Source: CAD feature listing. Evaluate the final solid. Frame: model axes, mm. A direction names the side the tool comes from. Round coordinates to 2 decimals unless told otherwise and drop trailing zeros. Order: outer loops, then holes, each group sorted by start corner. A loop starts at its lowest first (then second) coordinate and runs counter-clockwise, first axis right, second up. Notation, with made-up numbers: (55.5, 10) -> (105.5, 10) arc R16 ccw to (105.5, 30) -> close; hole circle Ø2 at (64.25, -7). An arc over 180 degrees is marked (long way). Write item = value, one per line. Start each with the question number.
(1) Ray query, line 1 (X direction, y = 0.05, z = 0); line 2 (Y direction, x = 2.25, z = 6.5). Return the intervals inside material, ascending.
(2) Reachability of faces 1 (the face through (-6, 14.15, -3)), 2 (the face through (-1.398, 3.549, 6.297)), 3 (the face through (1, -2, -3)) from +Z, -Z, +X, -X, +Y, -Y: full face, straight path, thin tool, end or side. Return the list, or none.
(3) Contact query for flat-ended pins moving along their axis: pin 1 Ø2 at (x, y) = (4, 14.5) entering from -Z; pin 2 Ø6 at (y, z) = (5.5, 4.5) entering from +X; pin 3 Ø1 at (y, z) = (3, -4.5) entering from +X. Output: stop coordinate, or through.
(4) Cut plane A-A on y = 12.5. Return the cut outline in (x, z), then the cut area to 3 significant figures.
(5) Draft query along X for faces 4 (the face through (2.111, -1.875, 4.059)), 5 (the face through (-0.35, 8.87, 1.56)), 6 (the face through (3, 7, -6)). Return one class per face: released by +X, released by -X, zero draft, split by the parting line, or undercut.
(6) Cut plane B-B on y = 9.25. Return the cut outline in (x, z).
Autodesk Inventor part; units mm, degrees
ref_plane "YZ Plane" through (0, 0, 0) normal (1, 0, 0) x (0, 1, 0)
ref_plane "XZ Plane" through (0, 0, 0) normal (0, 1, 0) x (-1, 0, 0)
ref_plane "XY Plane" through (0, 0, 0) normal (0, 0, 1) x (1, 0, 0)
sketch "Sketch1" plane through (0, 0, 0) normal (0, 0, 1) x (1, 0, 0)
  line L0 (0, 0) -> (0, 8.9988) construction
  line L1 (0, 0) -> (7.1408, 0) construction
  line L2 (0.9, 0) -> (2.3166, 18)
  line L3 (0.9, 0) -> (6.45, 0)
  line L4 (6.45, 0) -> (6.45, 7)
  line L5 (6.45, 7) -> (8, 7)
  line L6 (6.5, 18) -> (2.3166, 18)
  line L7 (6.5, 18) -> (5.85, 18)
  line L8 (5.85, 18) -> (5.85, 15)
  line L9 (5.85, 15) -> (6.5, 15)
  line L10 (6.5, 15) -> (6.5, 18)
  line L11 (5.85, 16.45) -> (5.3, 18)
  circle A0 centre (6.5, 15) radius 0.85
  line L12 (8, 7) -> (8, 14.15)
  line L13 (8, 14.15) -> (6.5, 14.15)
  line L14 (6.5, 14.15) -> (6.5, 15)
  point P0 (5.85, 15.5477)
  point P1 (6.5, 14.15)
  dimension "d0" = 7
  dimension "d1" = 6.45
  dimension "d4" = 18
  dimension "d6" = 4.5
  dimension "d7" = 0.9
  dimension "d9" = 1.7
  dimension "d10" = 3
  dimension "d11" = 0.55
  dimension "d12" = 1.55
  dimension "d18" = 6.5
  dimension "d19" = 0.65
  dimension "d20" = 8
revolve "Revolution1" add sketch "Sketch1" angle 360 about axis through (0, 0, 0) along (0, 1, 0) contours L2 L6 L11 L8 A0 L13 L12 L5 L4 L3
chamfer "Chamfer1" distance 0.5 angle 45 3 edges at (-8, 7, 0) (-2.3166, 18, 0) (-8, 14.15, 0)
fillet "Fillet1" radius 2 2 edges at (-5.85, 15.5477, 0) (-5.85, 16.45, 0)
sketch "Sketch2" plane through (0, 0, 0) normal (0, -1, 0) x (1, 0, 0)
  circle A0 centre (0, 0) radius 6.45
  circle A1 centre (0, 0) radius 0.9
extrude "Extrusion1" add sketch "Sketch2" along normal blind 2
chamfer "Chamfer2" distance 2 angle 45 2 edges at (-0.9, -2, 0) (-6.45, -2, 0)
properties part number "pipettetip_alignmenttool_v2"
Evaluation:
q1.line_1 = -6.45 to -0.9, 0.9 to 6.45
q1.line_2 = 7 to 14.15
q2.face_1 = +Y
q2.face_2 = -Y
q2.face_3 = +Z, -Z, +X, -X, -Y
q3.pin_1 = -7.21
q3.pin_2 = 7.67
q3.pin_3 = 5.06
q4.outline = circle Ø16 at (0, 0); hole circle Ø3.77 at (0, 0)
q4.area = 190 mm^2
q5.face_4 = split by the parting line
q5.face_5 = undercut
q5.face_6 = zero draft
q6.outline = circle Ø16 at (0, 0); hole circle Ø3.26 at (0, 0)
